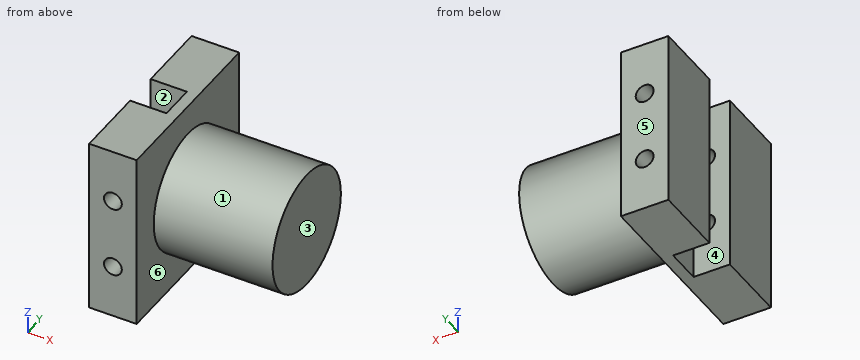
```python
from build123d import *

# Parameters (mm, degrees)
BOSS_EXTRUDE1_DEPTH = 15
SKETCH2_R           = 1.5
CUT_EXTRUDE1_DEPTH  = 35.481879299
SKETCH3_R           = 10
BOSS_EXTRUDE2_DEPTH = 20


with BuildPart() as part:
    # Sketch1 → Boss-Extrude1 (new, symmetric)
    with BuildSketch(Plane.XY):
        Polygon((0, -15), (0, 15), (-8, 15), (-8, 3), (-1.885714286, 3), (-1.885714286, -3), (-8, -3), (-8, -15), align=None)
    extrude(amount=BOSS_EXTRUDE1_DEPTH, both=True)

    # Sketch2 → Cut-Extrude1 (cut, through all)
    with BuildSketch(Plane(origin=(0, 15, 0), x_dir=(1, 0, 0), z_dir=(0, 1, 0))):
        with Locations(Location((-4, 6, 0), (0, 0, 270))):
            Circle(SKETCH2_R)
        with Locations((-4, -6)):
            Circle(SKETCH2_R)
    extrude(amount=-CUT_EXTRUDE1_DEPTH, mode=Mode.SUBTRACT)

    # Sketch3 → Boss-Extrude2 (add)
    with BuildSketch(Plane(origin=(0, 0, 0), x_dir=(0, 0, -1), z_dir=(1, 0, 0))):
        with Locations(Location((0, 0, 0), (0, 0, 90))):
            Circle(SKETCH3_R)
    extrude(amount=BOSS_EXTRUDE2_DEPTH)


solid = part.part
```
Here's how the part is built. I have some questions about the finished solid (model axes, mm). Face numbers are marked on the shaded views. A direction names the side the tool comes from. Round coordinates to 2 decimals unless told otherwise and drop trailing zeros. Write each loop counter-clockwise with the first axis right and the second up, starting at its lowest first coordinate (ties: lowest second). Pieces come first, ordered by that corner, then holes. Notation, with made-up numbers: M 50,-9.75 L 106,-9.75 A18 cw 106,17.25 Z; hole C 39.5,50 d10. An arc over 180 degrees is marked long. Answer as CSV lines item,"result". Start each with the question number.
1. I need wall thicknesses on probe 1 along X at (y, z) = (-12, -6); probe 2 along Y at (x, z) = (-4, 13.5); probe 3 along X at (y, z) = (5.75, 13.25). Which ranges of each line are inside material? Lowest first, please.
2. Suppose I cut it at C-C on y = 12.5. Write out the boundary of the cut face in (x, z), then the cut area to 3 significant figures.
3. Thinking about a two-plate mould opening in Y: for the marked faces 4, 5 and 6, which applies, released by +Y, released by -Y, zero draft, split by the parting line, or undercut?
4. On a 3-axis mill with a long thin cutter (end or side, diameter ignored), from which of +Z, -Z, +X, -X, +Y, -Y can I reach the whole of each face in a straight line? I mean the marked faces 1, 2 and 3. Say none if no direction works.
5. Suppose I cut it at A-A on x = -4. Write out the boundary of the cut face in (y, z), then the cut area to 3 significant figures.
6. Suppose I cut it at D-D on z = 11.5. Write out the boundary of the cut face in (x, y), then the cut area to 3 significant figures.
7. Suppose I cut it at B-B on z = 6. Write out the boundary of the cut face in (x, y), then the cut area to 3 significant figures.
8. I'm going to push flat-ended pins straight in: pin 1 Ø1.8 at (x, z) = (-4, -6) entering from +Y; pin 2 Ø4 at (x, z) = (8.5, 7) entering from +Y; pin 3 Ø8 at (x, y) = (5, 10) entering from -Z; pin 4 Ø4 at (x, z) = (16, -9.5) entering from -Y. Where does each tip first touch, or does it pass through?
Check result:
1,probe 1,"x = -8 to -5.5, -2.5 to 0"
1,probe 2,"y = -15 to -3, 3 to 15"
1,probe 3,"x = -8 to 0"
2,outline,"M -8,-15 L 0,-15 L 0,15 L -8,15 Z; hole C -4,-6 d3; hole C -4,6 d3"
2,area,"226 mm2"
3,face 4,"undercut"
3,face 5,"released by +Y"
3,face 6,"zero draft"
4,face 1,"+X"
4,face 2,"+Z, -Z, -X"
4,face 3,"+Z, -Z, +X, +Y, -Y"
5,outline,"M -15,-15 L -3,-15 L -3,-7.5 L -15,-7.5 Z; M -15,-4.5 L -3,-4.5 L -3,4.5 L -15,4.5 Z; M -15,7.5 L -3,7.5 L -3,15 L -15,15 Z; M 3,-15 L 15,-15 L 15,-7.5 L 3,-7.5 Z; M 3,-4.5 L 15,-4.5 L 15,4.5 L 3,4.5 Z; M 3,7.5 L 15,7.5 L 15,15 L 3,15 Z"
5,area,"576 mm2"
6,outline,"M -8,-15 L 0,-15 L 0,15 L -8,15 L -8,3 L -1.89,3 L -1.89,-3 L -8,-3 Z"
6,area,"203 mm2"
7,outline,"M -8,-15 L -5.5,-15 L -5.5,-3 L -8,-3 Z; M -8,3 L -5.5,3 L -5.5,15 L -8,15 Z; M -2.5,-15 L 0,-15 L 0,-8 L 20,-8 L 20,8 L 0,8 L 0,15 L -2.5,15 L -2.5,3 L -1.89,3 L -1.89,-3 L -2.5,-3 Z"
7,area,"451 mm2"
8,pin 1,"passes through"
8,pin 2,"stops at y = 8.66"
8,pin 3,"stops at z = -8"
8,pin 4,"stops at y = -6.61"
